Input: dimensioned drawing with shaded views. Units: mm. Origin: part minimum x, y, z. A direction names the side the tool comes from. Round coordinates to 2 decimals unless told otherwise and drop trailing zeros. Order: outer loops, then holes, each group sorted by start corner. A loop starts at its lowest first (then second) coordinate and runs counter-clockwise, first axis right, second up. Notation, with made-up numbers: (-16, -1) - (19, -1) arc R13 cw to (19, 3) - close; hole circle Ø3 at (74.5, -23.75). An arc over 180 degrees is marked (long way). One line per item, written item: value. Start each with the question number.
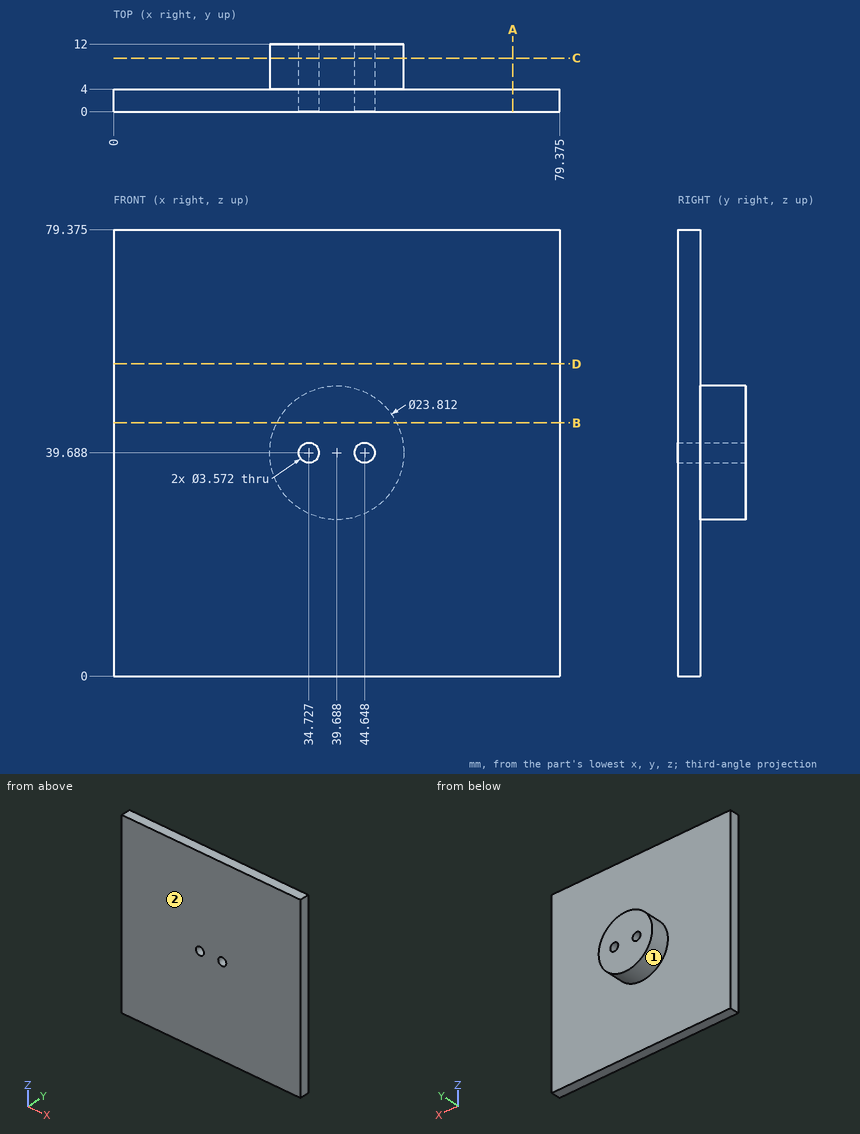
1. Section A-A (x = 71). Return the cut outline in (y, z) (1 decimal).
2. Pin query (flat end, axial travel): pin 1 (4.5 mm diameter, centred on x = 34.73, z = 39.69, fed in from +Y); pin 2 (1.5 mm diameter, centred on y = 6, z = 67, fed in from +X); pin 3 (1.5 mm diameter, centred on x = 69, z = 24, fed in from +Y); pin 4 (5 mm diameter, centred on x = 39.5, y = 8, fed in from +Z). Return the tip coordinate at first contact, or that it passes through.
3. Section B-B (z = 45). Return the cut outline in (x, y) (1 decimal), then the cut area to 3 significant figures.
4. Set-up query: the marked faces 1 and 2. Return all of +Z, -Z, +X, -X, +Y, -Y with unobstructed straight access to the full face (end or side cutting, diameter ignored); none if empty.
5. Line query: line 1 (Y direction, x = 73.5, z = 4); line 2 (Z direction, x = 42, y = 10.25); line 3 (Z direction, x = 36, y = 2.25) (1 decimal). Output: solid intervals per line, ascending. Write a range as from..to.
6. Section D-D (z = 55.5). Return the cut outline in (x, y) (1 decimal).
7. Section C-C (y = 9.5). Return the cut outline in (x, z) (1 decimal), then the cut area to 3 significant figures.
Solved:
1. outline: (0, 0) - (4, 0) - (4, 79.4) - (0, 79.4) - close
2. pin 1: stops at y = 12
2. pin 2: passes through
2. pin 3: stops at y = 4
2. pin 4: stops at z = 51.59
3. outline: (0, 0) - (79.4, 0) - (79.4, 4) - (50.3, 4) - (50.3, 12) - (29, 12) - (29, 4) - (0, 4) - close
3. area: 488 mm²
4. face 1: +Y
4. face 2: +Z, -Z, +X, -X, -Y
5. line 1: y = 0..4
5. line 2: z = 28.01..51.37
5. line 3: z = 0..38.4, 40.9..79.4
6. outline: (0, 0) - (79.4, 0) - (79.4, 4) - (0, 4) - close
7. outline: circle Ø23.8 at (39.7, 39.7); hole circle Ø3.6 at (34.7, 39.7); hole circle Ø3.6 at (44.6, 39.7)
7. area: 425 mm²
